from build123d import *

# Parameters (mm, degrees)
RACCORDO1_R = 1


with BuildPart() as part:
    # Schizzo1 → Rivoluzione1 (revolve)
    with BuildSketch(Plane.XY, mode=Mode.PRIVATE) as rivoluzione1_sk:
        with BuildLine():
            Line((-71, 0), (-73, 0))
            Line((-73, 0), (-73, 15))
            Line((-73, 15), (-69, 15))
            Line((-69, 15), (-69, 16))
            ThreePointArc((-69, 16), (-59.483339502, 25.516660498), (-46.483339502, 29))
            Line((-46.483339502, 29), (-16, 29))
            Line((-16, 29), (-20.618802154, 21))
            Line((-20.618802154, 21), (-46.483339502, 21))
            ThreePointArc((-46.483339502, 21), (-59.726832166, 16.773781497), (-68.074288586, 5.657532485))
            Line((-68.074288586, 5.657532485), (-69, 3))
            Line((-69, 3), (-71, 3))
            Line((-71, 3), (-71, 0))
        make_face()
    revolve(rivoluzione1_sk.sketch.rotate(Axis((0, 0, 0), (0, 1, 0)), 270), axis=Axis((0, 0, 0), (0, 1, 0)))

    # Raccordo1
    raccordo1_edges = [part.edges().sort_by_distance(p)[0] for p in [
        (0, 15, 69),
    ]]
    fillet(raccordo1_edges, radius=RACCORDO1_R - 0.0001)  # a hair under: the kernel refuses the full size


solid = part.part
For this review, take the finished solid that the model builds, in its own axes (mm). A direction names the side the tool comes from. Round coordinates to 2 decimals unless told otherwise and drop trailing zeros. Order: outer loops, then holes, each group sorted by start corner. A loop starts at its lowest first (then second) coordinate and runs counter-clockwise, first axis right, second up. Notation, with made-up numbers: M 54,45.25 L 91,45.25 A22 ccw 91,72.25 Z; hole C 87.25,87.5 d2. An arc over 180 degrees is marked long. Write each question's results on one line, items separated by ' | '. Start each with the question number.
1. Tool access review of faces 1 (the face through (-1, 29, -20)), 2 (the face through (62.99, 1.48, -32.76)): name each direction out of +Z, -Z, +X, -X, +Y, -Y from which nothing blocks a thin tool from reaching the whole face with its end or side.
2. To check wall thickness, follow L1, parallel to X at y = 1.7, z = 0; L2, parallel to Z at x = 19.5, y = 1.5; L3, parallel to Z at x = 26, y = 7.75. State the ranges of each line that lie inside material, in increasing order. Write a range as [from, to].
3. Add section C-C (y = 7.5). State the section outline as (x, z) points.
4. Draft analysis for pull direction X (two halves, no side actions). For faces 3 (the face through (71.264, 7.605, 15.825)), 4 (the face through (59, 15, -38)), 5 (the face through (-20.465, 5.491, -64.986)), state which applies: pulls with the +X half, pulls with the -X half, needs draft (parallel to the pull), parting line crosses it, or undercut.
5. Clearance check with flat-ended pins moving along their axes: pin 1 Ø1 at (x, z) = (-7, 44) entering from -Y; pin 2 Ø2 at (x, y) = (31.5, 20) entering from +Z; pin 3 Ø1 at (y, z) = (22.5, -2.5) entering from -X; pin 4 Ø3 at (x, z) = (-22, 41.5) entering from +Y. State where each tip first meets the part, or that it passes through.
Output values:
1) face 1: +Z, -Z, +X, -X, +Y | face 2: -Y
2) L1: [-73, -71], [71, 73] | L2: [-70.35, -68.27], [68.27, 70.35] | L3: [-68.21, -62], [62, 68.21]
3) outline: C 0,0 d146; hole C 0,0 d134.68
4) face 3: parting line crosses it | face 4: needs draft | face 5: undercut
5) pin 1: y = 21 | pin 2: z = 59.25 | pin 3: x = -64.18 | pin 4: y = 29
